Verification items for the finished model (mm, model axes). Face numbers are marked on the shaded views. A direction names the side the tool comes from. Give positions to 0.01 mm unless a question says otherwise; leave off trailing zeros. Write each loop counter-clockwise with the first axis right and the second up, starting at its lowest first coordinate (ties: lowest second). Pieces come first, ordered by that corner, then holes. Notation, with made-up numbers: (77, 76.5) - (103, 76.5) arc R22 cw to (103, 83.5) - close; hole circle Ø3 at (-30, -14.75). An arc over 180 degrees is marked (long way). Answer as a JSON object with one key per item and string values. Group by question number.
Item 1: Scan lines: line 1 along Y through (x, z) = (2.5, 15); line 2 along Z through (x, y) = (2, 0); line 3 along Y through (x, z) = (4.5, -5). Record each from-to range of solid material in increasing order. Write a range as [from, to].
Item 2: Tool access check on the marked faces 5 and 6. Record the directions out of +Z, -Z, +X, -X, +Y, -Y that give a thin tool (end or side, any length) a straight path to the whole face; none if there is none.
Item 3: Sectioned sample at B-B, the plane z = -7. Record the boundary of the cut face in (x, y), and give its area (3 significant figures).
Item 4: Draft check along Z on the marked faces 1, 2, 3 and 4. Enter one of: +Z half, -Z half, draft (parallel to the pull), parting line (faces both ways), or undercut.
Item 5: Sectioned sample at C-C, the plane y = 0. Record the boundary of the cut face in (x, z), and give its area (3 significant figures).
Item 6: Sectioned sample at D-D, the plane y = -28.5. Record the boundary of the cut face in (x, z).
Item 7: Sectioned sample at A-A, the plane x = 1.75. Record the boundary of the cut face in (y, z), and give its area (3 significant figures).
Item 8: Go/stop test with a flat-tipped pin: pin 1 (3 mm diameter, centred on x = 3.5, z = 24, fed in from +Y). Record where the tip stops, or that it passes through.
```python
from build123d import *

# Parameters (mm, degrees)
F1_DEPTH = 7
F2_DEPTH = 7
F3_DEPTH = 7
F0_R     = 10.5
F4_DEPTH = 7


with BuildPart() as f1:
    # F0 (on Right) → F1 (new body)
    with BuildSketch(Plane.YZ):
        with BuildLine():
            ThreePointArc((14.589096, -4.427731), (11.941496, -9.478775), (7.623098, -13.203594))
            ThreePointArc((7.623098, -13.203594), (12.978421, -33.004131), (12.030362, -53.494177))
            ThreePointArc((12.030362, -53.494177), (20.732247, -29.348026), (14.589096, -4.427731))
        make_face()
    extrude(amount=F1_DEPTH)



with BuildPart() as f2:
    # F0 (on Right) → F2 (new body)
    with BuildSketch(Plane.YZ):
        with BuildLine():
            ThreePointArc((-15.246197, 0), (-35.071627, 5.262423), (-52.342497, 16.328489))
            ThreePointArc((-52.342497, 16.328489), (-35.78226, -3.28064), (-11.129076, -10.420662))
            ThreePointArc((-11.129076, -10.420662), (-14.179608, -5.602251), (-15.246197, 0))
        make_face()
    extrude(amount=F2_DEPTH)


with BuildPart() as f3:
    # F0 (on Right) → F3 (new body)
    with BuildSketch(Plane.YZ):
        with BuildLine():
            ThreePointArc((40.312135, 37.165687), (15.050012, 32.628666), (-3.46002, 14.848393))
            ThreePointArc((-3.46002, 14.848393), (2.238112, 15.081027), (7.623098, 13.203594))
            ThreePointArc((7.623098, 13.203594), (22.093206, 27.741708), (40.312135, 37.165687))
        make_face()
    extrude(amount=F3_DEPTH)


with BuildPart() as f1_1:
    add(f1.part)

    add(f2.part)  # F4 merges F2

    add(f3.part)  # F4 merges F3
    # F0 (on Right) → F4 (join)
    with BuildSketch(Plane.YZ):
        with BuildLine():
            ThreePointArc((-3.46002, 14.848393), (-11.941496, 9.478775), (-15.246197, 0))
            ThreePointArc((-15.246197, 0), (-14.179608, -5.602251), (-11.129076, -10.420662))
            ThreePointArc((-11.129076, -10.420662), (-2.238112, -15.081027), (7.623098, -13.203594))
            ThreePointArc((7.623098, -13.203594), (11.941496, -9.478775), (14.589096, -4.427731))
            ThreePointArc((14.589096, -4.427731), (15.081027, -2.238112), (15.246197, 0))
            ThreePointArc((15.246197, 0), (13.203594, 7.623098), (7.623098, 13.203594))
            ThreePointArc((7.623098, 13.203594), (2.238112, 15.081027), (-3.46002, 14.848393))
        make_face()
        Circle(F0_R, mode=Mode.SUBTRACT)
    extrude(amount=F4_DEPTH)


solid = f1_1.part
```
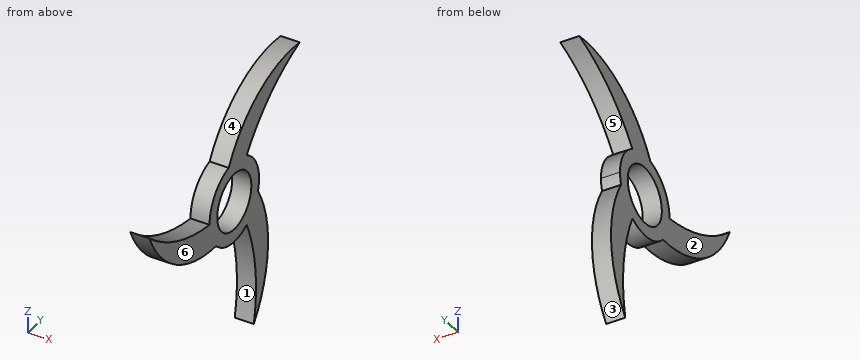
Geometry check:
{
 "1": {"line 1": "[-51.74, -50.8], [-3.37, 8.97]", "line 2": "[-15.25, -10.5], [10.5, 20.1]", "line 3": "[-32.9, -9.23], [9.23, 14.92]"},
 "2": {"face 5": "+X, -X, +Y", "face 6": "+Z, -Z, +X, +Y, -Y"},
 "3": {"outline": "(0, -28.74) - (7, -28.74) - (7, -7.83) - (0, -7.83) - close; (0, 7.83) - (7, 7.83) - (7, 16) - (0, 16) - close", "area": "204 mm^2"},
 "4": {"face 1": "undercut", "face 2": "draft", "face 3": "undercut", "face 4": "+Z half"},
 "5": {"outline": "(0, -15.25) - (7, -15.25) - (7, -10.5) - (0, -10.5) - close; (0, 10.5) - (7, 10.5) - (7, 20.1) - (0, 20.1) - close", "area": "100 mm^2"},
 "6": {"outline": "(0, -7.1) - (7, -7.1) - (7, 2.78) - (0, 2.78) - close"},
 "7": {"outline": "(-52.34, 16.33) arc R44.32 ccw to (-11.13, -10.42) arc R15.25 ccw to (7.62, -13.2) arc R66.35 cw to (12.03, -53.49) arc R44.32 ccw to (14.59, -4.43) arc R15.25 ccw to (15.25, 0) arc R15.25 ccw to (7.62, 13.2) arc R66.35 cw to (40.31, 37.17) arc R44.32 ccw to (-3.46, 14.85) arc R15.25 ccw to (-15.25, 0) arc R66.35 cw to start; hole circle Ø21 at (0, 0)", "area": "1,320 mm^2"},
 "8": {"pin 1": "y = 19.21"}
}
